Source: three-view drawing plus pictorial views. Frame: mm from the lowest corner of the part. A direction names the side the tool comes from. Round coordinates to 2 decimals unless told otherwise and drop trailing zeros. Write each loop counter-clockwise with the first axis right and the second up, starting at its lowest first coordinate (ties: lowest second). Pieces come first, ordered by that corner, then holes. Notation, with made-up numbers: M 20.5,49.25 L 36.5,49.25 A30 cw 36.5,82.25 Z; hole C 64.25,-2 d7. An arc over 180 degrees is marked long. Answer in a Markdown table with one row per item.
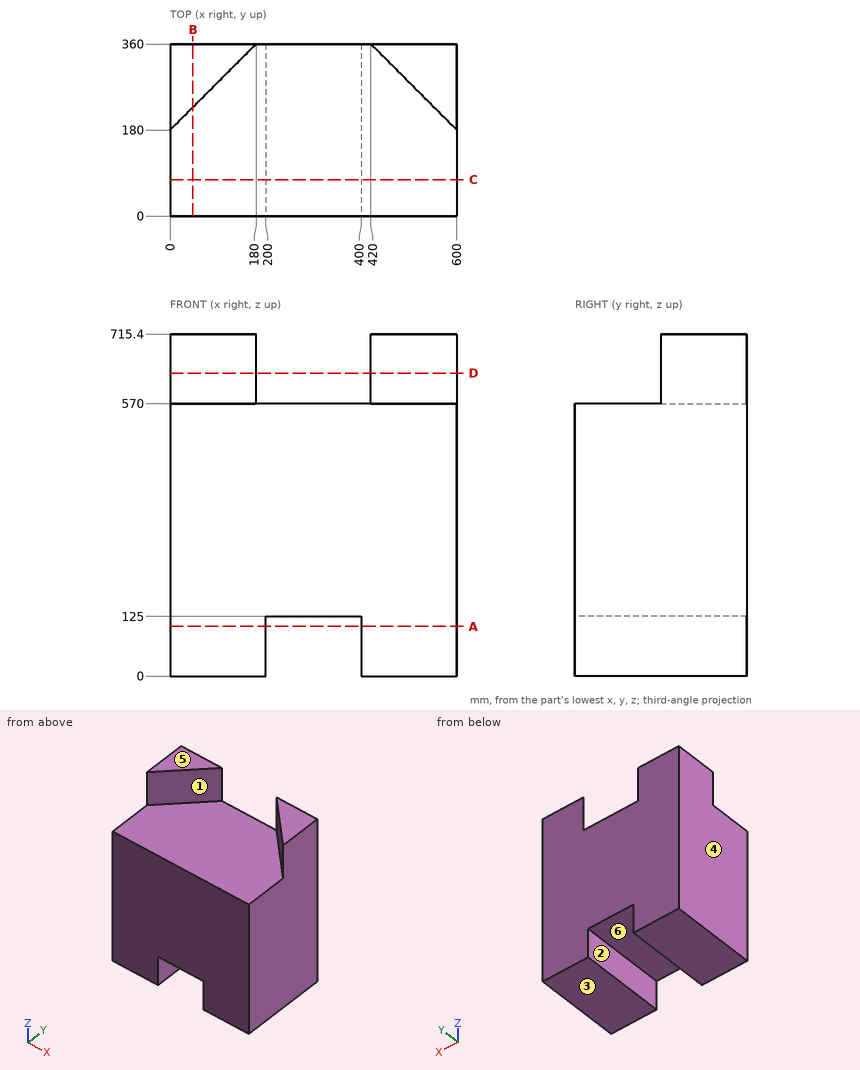
Q1. Section B-B (x = 47.5). Return loops of the section in (y, z), and give its area (3 significant figures).
Solutions:
| item | result |
|---|---|
| outline | M 0,0 L 360,0 L 360,715.4 L 227.5,715.4 L 227.5,570 L 0,570 Z |
| area | 224,000 mm2 |
Q2. Access query for the marked faces 1, 2 and 3. Directions: +Z, -Z, +X, -X, +Y, -Y. A direction counts if a zero-diameter tool reaches every point of the face in a straight line with its end or side. Return the directions, or none.
Solutions:
| item | result |
|---|---|
| face 1 | +Z, -Y |
| face 2 | -Z, +Y, -Y |
| face 3 | -Z, +X, -X, +Y, -Y |
Q3. Pull-direction query (X, two-part tool) for the marked faces 4, 5 and 6; classes: pulls with the +X half, pulls with the -X half, needs draft (parallel to the pull), parting line crosses it, or undercut.
Solutions:
| item | result |
|---|---|
| face 4 | pulls with the -X half |
| face 5 | needs draft |
| face 6 | undercut |
Q4. Section A-A (z = 104). Return loops of the section in (x, y), and give its area (3 significant figures).
Solutions:
| item | result |
|---|---|
| outline | M 0,0 L 200,0 L 200,360 L 0,360 Z; M 400,0 L 600,0 L 600,360 L 400,360 Z |
| area | 144,000 mm2 |
Q5. Section C-C (y = 76.5). Return loops of the section in (x, z).
Solutions:
| item | result |
|---|---|
| outline | M 0,0 L 200,0 L 200,125 L 400,125 L 400,0 L 600,0 L 600,570 L 0,570 Z |
Q6. Section D-D (z = 633.5). Return loops of the section in (x, y), and give its area (3 significant figures).
Solutions:
| item | result |
|---|---|
| outline | M 0,180 L 180,360 L 0,360 Z; M 420,360 L 600,180 L 600,360 Z |
| area | 32,400 mm2 |
Q7. Material intervals for probe 1 along X at (y, z) = (244, 97); probe 2 along Z at (x, y) = (321, 30); probe 3 along Z at (x, y) = (39, 181), sorted ascending.
Solutions:
| item | result |
|---|---|
| probe 1 | x = 0 to 200, 400 to 600 |
| probe 2 | z = 125 to 570 |
| probe 3 | z = 0 to 570 |
Q8. Contact query for a flat-ended pin moving along its axis: pin 1 Ø12 at (x, y) = (88.5, 226.5) entering from +Z. Output: stop coordinate, or through.
Solutions:
| item | result |
|---|---|
| pin 1 | stops at z = 570 |
